Can you work these out from the model? Positions are in its coordinate system, mm. Round coordinates to 2 decimals unless told otherwise and drop trailing zeros. Loops run counter-clockwise (first coordinate to the right, second up) from the corner with the lowest first, then second, coordinate; pieces in that order, holes last.
from build123d import *

# Parameters (mm, degrees)
SKETCH_1_R      = 4
EXTRUDE_1_DEPTH = 1


with BuildPart() as part:
    # 草图1 → 凸台-拉伸1 (new body)
    with BuildSketch(Plane.XY):
        with BuildLine():
            Line((-23.5, 31.5), (23.5, 31.5))
            ThreePointArc((23.5, 31.5), (29.156854249, 29.156854249), (31.5, 23.5))
            Line((31.5, 23.5), (31.5, -23.5))
            ThreePointArc((31.5, -23.5), (29.156854249, -29.156854249), (23.5, -31.5))
            Line((23.5, -31.5), (-23.5, -31.5))
            ThreePointArc((-23.5, -31.5), (-29.156854249, -29.156854249), (-31.5, -23.5))
            Line((-31.5, -23.5), (-31.5, 23.5))
            ThreePointArc((-31.5, 23.5), (-29.156854249, 29.156854249), (-23.5, 31.5))
        make_face()
        with Locations((-22.5, 22.5)):
            Circle(SKETCH_1_R, mode=Mode.SUBTRACT)
        with Locations(Location((22.5, 22.5, 0), (0, 0, 180))):
            Circle(SKETCH_1_R, mode=Mode.SUBTRACT)
        with Locations((22.5, -22.5)):
            Circle(SKETCH_1_R, mode=Mode.SUBTRACT)
        with Locations(Location((-22.5, -22.5, 0), (0, 0, 180))):
            Circle(SKETCH_1_R, mode=Mode.SUBTRACT)
        with Locations((0, 15.5)):
            Circle(SKETCH_1_R, mode=Mode.SUBTRACT)
    extrude(amount=EXTRUDE_1_DEPTH)


solid = part.part
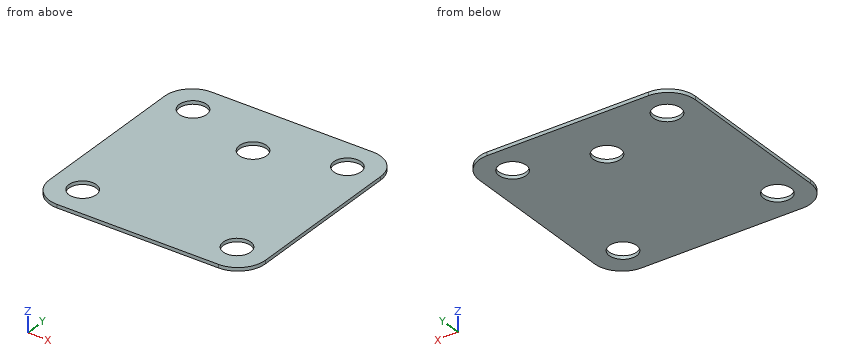
(1) If we section it at B-B, the plane y = 22.5: List the corners of the cut face in (x, z) for me, then the cut area to 3 significant figures.
Worked answers:
outline: (-31.5, 0) - (-26.5, 0) - (-26.5, 1) - (-31.5, 1) - close; (-18.5, 0) - (18.5, 0) - (18.5, 1) - (-18.5, 1) - close; (26.5, 0) - (31.5, 0) - (31.5, 1) - (26.5, 1) - close
area: 47.0 mm2
(2) If we section it at A-A, the plane x = 0: List the corners of the cut face in (y, z) for me, then the cut area to 3 significant figures.
Worked answers:
outline: (-31.5, 0) - (11.5, 0) - (11.5, 1) - (-31.5, 1) - close; (19.5, 0) - (31.5, 0) - (31.5, 1) - (19.5, 1) - close
area: 55.0 mm2
(3) Will this pin go through, and if not, where does the flat tip stop? P1, Ø7, axis at x = 0, y = 15.5, coming from the +Z side.
Worked answers:
P1: passes through
(4) If I drill on line 1 (Y direction, x = -22.5, z = 0.4); line 2 (Y direction, x = -23.5, z = 0.75); line 3 (X direction, y = 17, z = 0.45), over which ranges is the centre line in solid material (lowest first)?
Worked answers:
line 1: y = -31.5 to -26.5, -18.5 to 18.5, 26.5 to 31.5
line 2: y = -31.5 to -26.37, -18.63 to 18.63, 26.37 to 31.5
line 3: x = -31.5 to -3.71, 3.71 to 31.5
(5) If we section it at C-C, the plane y = 15.5: List the corners of the cut face in (x, z) for me.
Worked answers:
outline: (-31.5, 0) - (-4, 0) - (-4, 1) - (-31.5, 1) - close; (4, 0) - (31.5, 0) - (31.5, 1) - (4, 1) - close
